Verification items for this drawing (mm, ordinates from the low corner). A direction names the side the tool comes from. Coordinates: 2 decimals unless noted, no trailing zeros. Order: outer loops, then holes, each group sorted by start corner. A loop starts at its lowest first (then second) coordinate and runs counter-clockwise, first axis right, second up. Notation, with made-up numbers: (0, -26) -> (13, -26) arc R19 cw to (13, -8) -> close; hole circle Ø11 at (10.25, -26). An arc over 180 degrees is marked (long way). Write item = value, one per line. Start each with the question number.
1. Thickness scan on line 1 along Z through (x, y) = (33.5, 15); line 2 along Y through (x, z) = (25, 9.75); line 3 along X through (y, z) = (3, 1). Record the ranges inside material, lowest first. Write a range as from..to.
2. Cross-section at B-B on z = 6.25. Record the cut outline in (x, y), plus the area to 3 significant figures.
3. Release check for a two-part mould opening along Y. For the marked faces 1, 2 and 3 record: +Y half, -Y half, draft (parallel to the pull), parting line (faces both ways), or undercut.
4. Cross-section at C-C on x = 25. Record the cut outline in (y, z).
5. Cross-section at D-D on y = 12.5. Record the cut outline in (x, z).
6. Cross-section at A-A on x = 35.5. Record the cut outline in (y, z), plus the area to 3 significant figures.
7. Go/stop test with flat-tipped pins: P1, Ø2, axis at x = 40.5, z = 5.5, coming from the +Y side; P2, Ø2, axis at y = 6.5, z = 5, coming from the -X side; P3, Ø4, axis at x = 36.5, y = 13, coming from the -Z side; P4, Ø6, axis at x = 8, y = 4.5, coming from the +Z side. Record where each tip stops, or that it passes through.
8. Set-up check for the marked faces 4, 5, 6 and 7: record each of +Z, -Z, +X, -X, +Y, -Y from which the full face is reachable in a straight line by a thin tool's end or side.
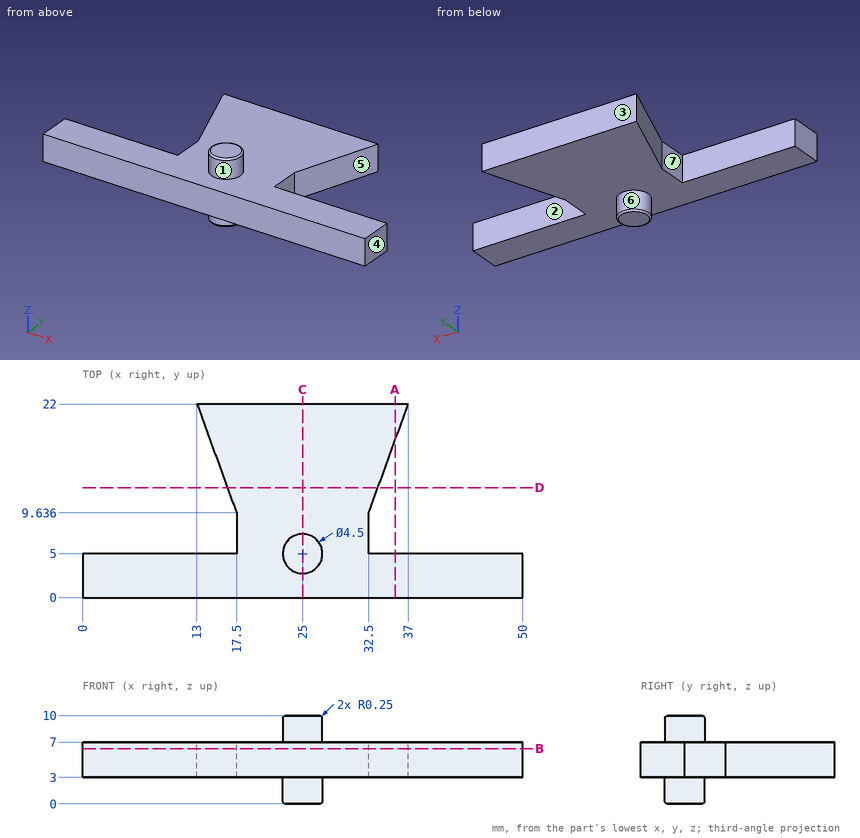
Worked out:
q1.line_1 = 3..7
q1.line_2 = 2.75..7.25
q1.line_3 = 23.97..26.03
q2.outline = (0, 0) -> (50, 0) -> (50, 5) -> (32.5, 5) -> (32.5, 9.64) -> (37, 22) -> (13, 22) -> (17.5, 9.64) -> (17.5, 5) -> (0, 5) -> close
q2.area = 561 mm²
q3.face_1 = parting line
q3.face_2 = undercut
q3.face_3 = +Y half
q4.outline = (0, 3) -> (2.75, 3) -> (2.75, 0.25) arc R0.25 ccw to (3, 0) -> (7, 0) arc R0.25 ccw to (7.25, 0.25) -> (7.25, 3) -> (22, 3) -> (22, 7) -> (7.25, 7) -> (7.25, 9.75) arc R0.25 ccw to (7, 10) -> (3, 10) arc R0.25 ccw to (2.75, 9.75) -> (2.75, 7) -> (0, 7) -> close
q5.outline = (16.46, 3) -> (33.54, 3) -> (33.54, 7) -> (16.46, 7) -> close
q6.outline = (0, 3) -> (5, 3) -> (5, 7) -> (0, 7) -> close; (17.88, 3) -> (22, 3) -> (22, 7) -> (17.88, 7) -> close
q6.area = 36.5 mm²
q7.P1 = 5
q7.P2 = 17.5
q7.P3 = through
q7.P4 = 7
q8.face_4 = +Z, -Z, +X, +Y, -Y
q8.face_5 = +Z, -Z, +X
q8.face_6 = -Z
q8.face_7 = +Z, -Z, -X
